```python
from build123d import *

# Parameters (mm, degrees)
SKETCH1_R           = 12
BOSS_EXTRUDE1_DEPTH = 30
SKETCH2_R           = 13.5
BOSS_EXTRUDE2_DEPTH = 27
SKETCH3_R           = 2.15
BOSS_EXTRUDE3_DEPTH = 7
FILLET1_R           = 2
SKETCH4_R           = 3.215
BOSS_EXTRUDE4_DEPTH = 2.32
FILLET2_R           = 2
SKETCH5_W           = 1.5
SKETCH5_H           = 2.3
BOSS_EXTRUDE5_DEPTH = 4.3


with BuildPart() as part:
    # Sketch1 → Boss-Extrude1 (new body)
    with BuildSketch(Plane(origin=(0, 0, 0), x_dir=(1, 0, 0), z_dir=(0, 1, 0))):
        Circle(SKETCH1_R)
    extrude(amount=BOSS_EXTRUDE1_DEPTH)

    # Sketch2 → Boss-Extrude2 (add)
    with BuildSketch(Plane(origin=(0, 30, 0), x_dir=(1, 0, 0), z_dir=(0, 1, 0))):
        Circle(SKETCH2_R)
    extrude(amount=BOSS_EXTRUDE2_DEPTH)

    # Sketch3 → Boss-Extrude3 (add)
    with BuildSketch(Plane(origin=(0, 57, 0), x_dir=(1, 0, 0), z_dir=(0, 1, 0))):
        Circle(SKETCH3_R)
    extrude(amount=BOSS_EXTRUDE3_DEPTH)

    # Fillet1
    fillet1_edges = [part.edges().sort_by_distance(p)[0] for p in [
        (-2.15, 64, 0),
    ]]
    fillet(fillet1_edges, radius=FILLET1_R)

    # Sketch4 → Boss-Extrude4 (add)
    with BuildSketch(Plane.XZ):
        Circle(SKETCH4_R)
    extrude(amount=BOSS_EXTRUDE4_DEPTH)

    # Fillet2
    fillet2_edges = [part.edges().sort_by_distance(p)[0] for p in [
        (-3.215, -2.32, 0),
    ]]
    fillet(fillet2_edges, radius=FILLET2_R)

    # Sketch5 → Boss-Extrude5 (add)
    with BuildSketch(Plane.XZ):
        with Locations((9.75, 0)):
            Rectangle(SKETCH5_W, SKETCH5_H)
        with Locations((-9.75, 0)):
            Rectangle(SKETCH5_W, SKETCH5_H)
    extrude(amount=BOSS_EXTRUDE5_DEPTH)


solid = part.part
```
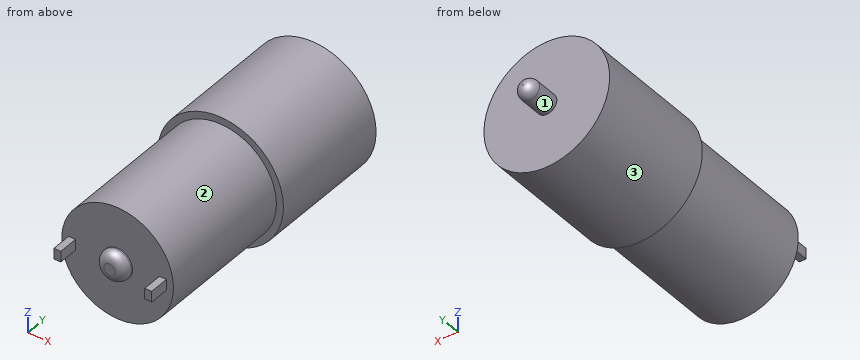
Model file for the job. Use its own axes, mm. Face numbers are marked on the shaded views. A direction names the side the tool comes from. Coordinates: 2 decimals unless noted, no trailing zeros. Order: outer loops, then holes, each group sorted by start corner. A loop starts at its lowest first (then second) coordinate and runs counter-clockwise, first axis right, second up. Notation, with made-up numbers: (-15.75, -23.75) - (16.25, -23.75) arc R25 cw to (16.25, -6.75) - close; hole circle Ø8 at (86.5, 72.25). An arc over 180 degrees is marked (long way). Return JSON: item names as keys, results as strings. Group by question number.
1) Flat gauge pins, fed straight in: P1, Ø1.2, axis at y = -2, z = 0.5, coming from the +X side; P2, Ø4, axis at x = -6.5, y = 27.5, coming from the -Z side; P3, Ø1.2, axis at x = 10, y = -1.5, coming from the +Z side. Where does each tip first touch, or does it go through?
2) Saw through at B-B, the plane y = 51. Write the cut outline in (x, z), plus the area to 3 significant figures.
3) Probe line 1 (Y direction, x = 9.5, z = 1); line 2 (Y direction, x = 6.75, z = 4.5); line 3 (Z direction, x = -10.5, y = 22). List the from-to ranges inside material, lowest first. Write a range as from..to.
4) Saw through at C-C, the plane x = -6. Write the cut outline in (y, z).
5) Saw through at A-A, the plane z = 6.25. Write the cut outline in (x, y), plus the area to 3 significant figures.
6) Saw through at D-D, the plane y = 26. Write the cut outline in (x, z), plus the area to 3 significant figures.
7) Tool access for the marked faces 1, 2 and 3: list every direction of +Z, -Z, +X, -X, +Y, -Y with a clear straight run to the whole face (end or side of a thin tool).
Values found:
{
 "1": {"P1": "stops at x = 10.5", "P2": "stops at z = -11.12", "P3": "stops at z = 1.15"},
 "2": {"outline": "circle Ø27 at (0, 0)", "area": "573 mm²"},
 "3": {"line 1": "y = -4.3..57", "line 2": "y = 0..57", "line 3": "z = -5.81..5.81"},
 "4": {"outline": "(0, -10.39) - (30, -10.39) - (30, -12.09) - (57, -12.09) - (57, 12.09) - (30, 12.09) - (30, 10.39) - (0, 10.39) - close"},
 "5": {"outline": "(-11.97, 30) - (-10.24, 30) - (-10.24, 0) - (10.24, 0) - (10.24, 30) - (11.97, 30) - (11.97, 57) - (-11.97, 57) - close", "area": "1,260 mm²"},
 "6": {"outline": "circle Ø24 at (0, 0)", "area": "452 mm²"},
 "7": {"face 1": "+Y", "face 2": "-Y", "face 3": "+Y, -Y"}
}
